from build123d import *

# Parameters (mm, degrees)
SKETCH1_W           = 50
SKETCH1_H           = 50
BOSS_EXTRUDE1_DEPTH = 50
SHELL1_T            = -3
FILLET1_R           = 2
SKETCH3_W           = 6
SKETCH3_H           = 6
BOSS_EXTRUDE2_DEPTH = 47
SKETCH4_R           = 1.25
CUT_EXTRUDE1_DEPTH  = 25
SKETCH5_R           = 10
CUT_EXTRUDE2_DEPTH  = 51
SKETCH8_W           = 22
SKETCH8_H           = 4
CUT_EXTRUDE4_DEPTH  = 51
SKETCH9_W           = 50
SKETCH9_H           = 9.65
CUT_EXTRUDE5_DEPTH  = 51


with BuildPart() as part:
    # Sketch1 → Boss-Extrude1 (new body)
    with BuildSketch(Plane(origin=(0, 0, 0), x_dir=(1, 0, 0), z_dir=(0, 1, 0))):
        Rectangle(SKETCH1_W, SKETCH1_H)
    extrude(amount=BOSS_EXTRUDE1_DEPTH)

    # Shell1
    shell1_openings = [part.faces().sort_by_distance(p)[0] for p in [
        (0, 0, 0),
    ]]
    offset(amount=SHELL1_T, openings=shell1_openings, kind=Kind.INTERSECTION)

    # Fillet1
    fillet1_edges = [part.edges().sort_by_distance(p)[0] for p in [
        (-25, 50, 0),
        (0, 50, 25),
        (25, 50, 0),
        (0, 50, -25),
        (25, 25, 25),
        (-25, 25, 25),
        (-25, 25, -25),
        (25, 25, -25),
    ]]
    fillet(fillet1_edges, radius=FILLET1_R)

    # Sketch3 → Boss-Extrude2 (add)
    with BuildSketch(Plane.XZ.offset(-47)):
        with Locations((19, 19)):
            Rectangle(SKETCH3_W, SKETCH3_H)
        with Locations((-19, 19)):
            Rectangle(SKETCH3_W, SKETCH3_H)
        with Locations((19, -19)):
            Rectangle(SKETCH3_W, SKETCH3_H)
        with Locations((-19, -19)):
            Rectangle(SKETCH3_W, SKETCH3_H)
    extrude(amount=BOSS_EXTRUDE2_DEPTH)

    # Sketch4 → Cut-Extrude1 (cut)
    with BuildSketch(Plane.XZ):
        with Locations((-19, 19)):
            Circle(SKETCH4_R)
        with Locations((19, 19)):
            Circle(SKETCH4_R)
        with Locations((19, -19)):
            Circle(SKETCH4_R)
        with Locations((-19, -19)):
            Circle(SKETCH4_R)
    extrude(amount=-CUT_EXTRUDE1_DEPTH, mode=Mode.SUBTRACT)

    # Sketch5 → Cut-Extrude2 (cut, through all)
    with BuildSketch(Plane(origin=(0, 50, 0), x_dir=(1, 0, 0), z_dir=(0, 1, 0))):
        Circle(SKETCH5_R)
    extrude(amount=-CUT_EXTRUDE2_DEPTH, mode=Mode.SUBTRACT)

    # Sketch8 → Cut-Extrude4 (cut, through all)
    with BuildSketch(Plane(origin=(0, 50, 0), x_dir=(1, 0, 0), z_dir=(0, 1, 0))):
        Rectangle(SKETCH8_W, SKETCH8_H)
    extrude(amount=-CUT_EXTRUDE4_DEPTH, mode=Mode.SUBTRACT)

    # Sketch9 → Cut-Extrude5 (cut, through all)
    with BuildSketch(Plane(origin=(0, 0, -25), x_dir=(-1, 0, 0), z_dir=(0, 0, -1))):
        with Locations((0, 4.825)):
            Rectangle(SKETCH9_W, SKETCH9_H)
    extrude(amount=-CUT_EXTRUDE5_DEPTH, mode=Mode.SUBTRACT)


solid = part.part
Work out the finished part from the listing and answer in its coordinate system (mm). A direction names the side the tool comes from. Coordinates: 2 decimals unless noted, no trailing zeros. Write each loop counter-clockwise with the first axis right and the second up, starting at its lowest first coordinate (ties: lowest second). Pieces come first, ordered by that corner, then holes.
1. Consider line 1 along Z through (x, y) = (19, 14.5); line 2 along X through (y, z) = (44.5, 7.5); line 3 along Z through (x, y) = (20.5, 15). Determine where each line is inside the solid, lowest interval first.
Results list:
line 1: z = -25 to -20.25, -17.75 to -16, 16 to 17.75, 20.25 to 25
line 2: x = -25 to -22, 22 to 25
line 3: z = -25 to -16, 16 to 25
2. The part is cut by section B-B, the plane z = -21. Write down the section's boundary in (x, y), and give its area (3 significant figures).
Results list:
outline: (-25, 9.65) - (-16, 9.65) - (-16, 47) - (16, 47) - (16, 9.65) - (25, 9.65) - (25, 48) arc R2 ccw to (23, 50) - (-23, 50) arc R2 ccw to (-25, 48) - close
area: 821 mm2
3. Flat-ended cylindrical pins translate along their axes: pin 1 (0.6 mm diameter, centred on x = 10.5, y = 49, fed in from +Z); pin 2 (1.2 mm diameter, centred on x = 19.5, z = -19, fed in from -Y); pin 3 (1.5 mm diameter, centred on y = 49, z = -1, fed in from -X); pin 4 (3 mm diameter, centred on x = 19, z = -19, fed in from -Y). Find the tip coordinate at first contact, or state that the pin passes through.
Results list:
pin 1: stops at z = 24.87
pin 2: stops at y = 25
pin 3: stops at x = -24.98
pin 4: stops at y = 9.65
4. The part is cut by section A-A, the plane y = 13. Write down the section's boundary in (x, z).
Results list:
outline: (-25, -23) arc R2 ccw to (-23, -25) - (23, -25) arc R2 ccw to (25, -23) - (25, 23) arc R2 ccw to (23, 25) - (-23, 25) arc R2 ccw to (-25, 23) - close; hole (-22, -16) - (-16, -16) - (-16, -22) - (16, -22) - (16, -16) - (22, -16) - (22, 16) - (16, 16) - (16, 22) - (-16, 22) - (-16, 16) - (-22, 16) - close; hole circle Ø2.5 at (-19, -19); hole circle Ø2.5 at (-19, 19); hole circle Ø2.5 at (19, -19); hole circle Ø2.5 at (19, 19)
5. For a pull along X with two mould halves and no side action, classify faces 4 (the flat face through (22.3, 9.65, -2)), 5 (the flat face through (19, 25, -19)), 6 (the cylindrical face through (-24.43, 49.4, -0.32)) as +X half, -X half, draft (parallel to the pull), parting line (faces both ways), or undercut.
Results list:
face 4: draft
face 5: undercut
face 6: -X half
6. For faces 1 (the flat face through (0, 28, 22)), 2 (the cylindrical face through (0, 49, 10)), 3 (the cylindrical face through (-24.43, 29.09, -24.4)), determine the directions among +Z, -Z, +X, -X, +Y, -Y from which every point of the face is accessible in a straight line to the end or side of a thin tool.
Results list:
face 1: -Y
face 2: +Y, -Y
face 3: -Z, -X, +Y, -Y
7. The part is cut by section D-D, the plane x = -17. Write down the section's boundary in (y, z), and give its area (3 significant figures).
Results list:
outline: (9.65, -25) - (48, -25) arc R2 ccw to (50, -23) - (50, 23) arc R2 ccw to (48, 25) - (9.65, 25) - (9.65, 16) - (47, 16) - (47, -16) - (9.65, -16) - close
area: 821 mm2
8. The part is cut by section C-C, the plane z = 8.5. Write down the section's boundary in (x, y), and give its area (3 significant figures).
Results list:
outline: (-25, 9.65) - (-22, 9.65) - (-22, 47) - (-5.27, 47) - (-5.27, 50) - (-23, 50) arc R2 ccw to (-25, 48) - close; (5.27, 47) - (22, 47) - (22, 9.65) - (25, 9.65) - (25, 48) arc R2 ccw to (23, 50) - (5.27, 50) - close
area: 341 mm2
